from build123d import *

# Parameters (mm, degrees)
SKETCH_1_W          = 75
SKETCH_1_H          = 60
EXTRUDE_1_DEPTH     = 4
SKETCH_2_R          = 2
CUT_EXTRUDE_1_DEPTH = 4
SKETCH_3_R          = 1.5
CUT_EXTRUDE_2_DEPTH = 49.189729196


with BuildPart() as part:
    # 草图1 → 凸台-拉伸1 (new body)
    with BuildSketch(Plane(origin=(0, 0, 0), x_dir=(1, 0, 0), z_dir=(0, 1, 0))):
        Rectangle(SKETCH_1_W, SKETCH_1_H)
    extrude(amount=EXTRUDE_1_DEPTH)

    # 草图2 → 切除-拉伸1 (cut)
    with BuildSketch(Plane(origin=(0, 0, 0), x_dir=(1, 0, 0), z_dir=(0, 1, 0))):
        with Locations(Location((7.5, 17.5, 0), (0, 0, 270))):
            Circle(SKETCH_2_R)
        with Locations(Location((7.5, 10.5, 0), (0, 0, 270))):
            Circle(SKETCH_2_R)
        with Locations(Location((7.5, 3.5, 0), (0, 0, 270))):
            Circle(SKETCH_2_R)
        with Locations(Location((7.5, -3.5, 0), (0, 0, 270))):
            Circle(SKETCH_2_R)
        with Locations(Location((7.5, -10.5, 0), (0, 0, 270))):
            Circle(SKETCH_2_R)
        with Locations(Location((7.5, -17.5, 0), (0, 0, 270))):
            Circle(SKETCH_2_R)
    extrude(amount=CUT_EXTRUDE_1_DEPTH, mode=Mode.SUBTRACT)

    # 草图3 → 切除-拉伸2 (cut, through all)
    with BuildSketch(Plane(origin=(0, 0, 0), x_dir=(1, 0, 0), z_dir=(0, 1, 0))):
        with Locations(Location((-32.5, 25, 0), (0, 0, 270))):
            Circle(SKETCH_3_R)
        with Locations(Location((32.5, 25, 0), (0, 0, 90))):
            Circle(SKETCH_3_R)
        with Locations(Location((32.5, -25, 0), (0, 0, 270))):
            Circle(SKETCH_3_R)
        with Locations(Location((-32.5, -25, 0), (0, 0, 90))):
            Circle(SKETCH_3_R)
        with Locations(Location((0, -25, 0), (0, 0, 90))):
            Circle(SKETCH_3_R)
        with Locations(Location((0, 25, 0), (0, 0, 270))):
            Circle(SKETCH_3_R)
    extrude(amount=CUT_EXTRUDE_2_DEPTH, mode=Mode.SUBTRACT)


solid = part.part
Geometry check sheet. Reference: the model listing, model coordinates, mm. Coordinates: 2 decimals unless noted, no trailing zeros. Order: outer loops, then holes, each group sorted by start corner. A loop starts at its lowest first (then second) coordinate and runs counter-clockwise, first axis right, second up. Notation, with made-up numbers: (4, 47) -> (27, 47) arc R18 cw to (27, 67) -> close; hole circle Ø4 at (-6.75, 26). An arc over 180 degrees is marked (long way). Use a Markdown table: item, result. Add a question column.
1. Material ranges on L1, parallel to X at y = 0.85, z = 25; L2, parallel to X at y = 1.95, z = -17.5; L3, parallel to X at y = 0.55, z = -24.5, recorded low to high.
2. Cross-section at A-A (x = -32.5). Enter the section's corners in (y, z).
3. Cross-section at D-D (z = -17.5). Enter the section's corners in (x, y), and give its area (3 significant figures).
4. Go/stop test with a flat-tipped pin: pin 1 Ø4 at (x, z) = (0, -25) entering from -Y. Record where the tip stops, or that it passes through.
5. Cross-section at C-C (y = 1.65). Give the number of separate pieces and of enclosed holes in the cut face, and give its area (3 significant figures).
6. Mould release check, pull along Z, two halves, no side actions. Record for faces 1 (the face through (-1, 2, -30)), 2 (the face through (-1, 2, 30)), 3 (the face through (0.07, 1.97, -26.5)): pulls with the +Z half, pulls with the -Z half, needs draft (parallel to the pull), parting line crosses it, or undercut.
7. Cross-section at B-B (z = 25). Enter the section's corners in (x, y).
Filled sheet:
| question | item | result |
|---|---|---|
| 1 | L1 | -37.5 to -34, -31 to -1.5, 1.5 to 31, 34 to 37.5 |
| 1 | L2 | -37.5 to 5.5, 9.5 to 37.5 |
| 1 | L3 | -37.5 to -33.91, -31.09 to -1.41, 1.41 to 31.09, 33.91 to 37.5 |
| 2 | outline | (0, -30) -> (4, -30) -> (4, -26.5) -> (0, -26.5) -> close; (0, -23.5) -> (4, -23.5) -> (4, 23.5) -> (0, 23.5) -> close; (0, 26.5) -> (4, 26.5) -> (4, 30) -> (0, 30) -> close |
| 3 | outline | (-37.5, 0) -> (5.5, 0) -> (5.5, 4) -> (-37.5, 4) -> close; (9.5, 0) -> (37.5, 0) -> (37.5, 4) -> (9.5, 4) -> close |
| 3 | area | 284 mm2 |
| 4 | pin 1 | y = 0 |
| 5 | separate pieces | 1 |
| 5 | enclosed holes | 12 |
| 5 | area | 4,380 mm2 |
| 6 | face 1 | pulls with the -Z half |
| 6 | face 2 | pulls with the +Z half |
| 6 | face 3 | undercut |
| 7 | outline | (-37.5, 0) -> (-34, 0) -> (-34, 4) -> (-37.5, 4) -> close; (-31, 0) -> (-1.5, 0) -> (-1.5, 4) -> (-31, 4) -> close; (1.5, 0) -> (31, 0) -> (31, 4) -> (1.5, 4) -> close; (34, 0) -> (37.5, 0) -> (37.5, 4) -> (34, 4) -> close |
